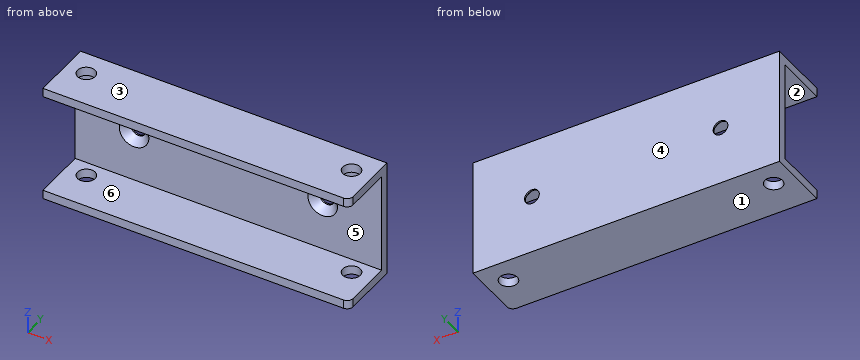
```python
from build123d import *

# Parameters (mm, degrees)
F0_W     = 104
F0_H     = 3
F1_DEPTH = 21
F0_H_2   = 34
F0_R     = 2.5
F2_DEPTH = 3
F4_D     = 6
F5_SIZE  = 2.5
F6_SIZE  = 2.5
F7_R     = 2


with BuildPart() as f1:
    # F0 (on Front) → F1 (new body)
    with BuildSketch(Plane.XZ):
        with Locations((0, 18.5)):
            Rectangle(F0_W, F0_H)
    extrude(amount=F1_DEPTH)



with BuildPart() as f1b:
    # F0 (on Front) → F1, piece 2 (new body)
    with BuildSketch(Plane.XZ):
        with Locations((0, -18.5)):
            Rectangle(F0_W, F0_H)
    extrude(amount=F1_DEPTH)


with BuildPart() as f1_1:
    add(f1.part)

    add(f1b.part)  # F2 merges F1b
    # F0 (on Front) → F2 (join)
    with BuildSketch(Plane.XZ):
        Rectangle(F0_W, F0_H_2)
        with Locations((-32, 0)):
            Circle(F0_R, mode=Mode.SUBTRACT)
        with Locations((32, 0)):
            Circle(F0_R, mode=Mode.SUBTRACT)
    extrude(amount=F2_DEPTH)

    # F4 (through all)
    with Locations(Plane(origin=(0, 0, -20), x_dir=(1, 0, 0), z_dir=(0, 0, -1))):
        with Locations((-45, 8.3), (45, 8.2999998429)):
            Hole(F4_D / 2)

    # F5
    f5_edges = [f1_1.edges().sort_by_distance(p)[0] for p in [
        (-34.5, -3, 0),
    ]]
    chamfer(f5_edges, length=F5_SIZE)

    # F6
    f6_edges = [f1_1.edges().sort_by_distance(p)[0] for p in [
        (29.5, -3, 0),
    ]]
    chamfer(f6_edges, length=F6_SIZE)

    # F7
    f7_edges = [f1_1.edges().sort_by_distance(p)[0] for p in [
        (52, -21, -18.5),
        (52, -21, 18.5),
    ]]
    fillet(f7_edges, radius=F7_R)


solid = f1_1.part
```
Read the model definition and answer for the solid it produces. Units are mm, in the model's axes. Face numbers are marked on the shaded views. A direction names the side the tool comes from. Coordinates: 2 decimals unless noted, no trailing zeros. Write each loop counter-clockwise with the first axis right and the second up, starting at its lowest first coordinate (ties: lowest second). Pieces come first, ordered by that corner, then holes. Notation, with made-up numbers: (4, -7.5) -> (8, -7.5) arc R29 ccw to (8, 12.5) -> close; hole circle Ø4 at (-35.75, -36.5). An arc over 180 degrees is marked (long way). Return JSON: item names as keys, results as strings.
1. Determine the mould class of the marked faces 3, 4, 5 and 6 for opening direction Z: pulls with the +Z half, pulls with the -Z half, needs draft (parallel to the pull), parting line crosses it, or undercut.
Found:
{"face 3": "pulls with the +Z half", "face 4": "needs draft", "face 5": "undercut", "face 6": "undercut"}
2. A tool of negligible diameter and unlimited length cuts with its end or side. For the marked faces 1 and 2, from which of +Z, -Z, +X, -X, +Y, -Y can it reach the whole face along a straight path? Write none if from no direction.
Found:
{"face 1": "-Z, +X, -X, +Y, -Y", "face 2": "+X, -X, -Y"}
3. A cutting plane is placed at D-D (y = -14). Determine the outline of the cut face in (x, z).
Found:
{"outline": "(-52, -20) -> (52, -20) -> (52, -17) -> (-52, -17) -> close; (-52, 17) -> (52, 17) -> (52, 20) -> (-52, 20) -> close"}
4. A cutting plane is placed at C-C (x = 32). Determine the outline of the cut face in (y, z), and give its area (3 significant figures).
Found:
{"outline": "(-21, -20) -> (0, -20) -> (0, -2.5) -> (-0.5, -2.5) -> (-3, -5) -> (-3, -17) -> (-21, -17) -> close; (-21, 17) -> (-3, 17) -> (-3, 5) -> (-0.5, 2.5) -> (0, 2.5) -> (0, 20) -> (-21, 20) -> close", "area": "207 mm2"}
5. A cutting plane is placed at A-A (z = 0). Determine the outline of the cut face in (x, y), and give its area (4 significant figures).
Found:
{"outline": "(-52, -3) -> (-37, -3) -> (-34.5, -0.5) -> (-34.5, 0) -> (-52, 0) -> close; (-29.5, -0.5) -> (-27, -3) -> (27, -3) -> (29.5, -0.5) -> (29.5, 0) -> (-29.5, 0) -> close; (34.5, -0.5) -> (37, -3) -> (52, -3) -> (52, 0) -> (34.5, 0) -> close", "area": "269.5 mm2"}
6. Each of these flat-tipped pins is pushed along its axis until it touches: P1, Ø3, axis at x = 22, z = 14, coming from the -Y side; P2, Ø6.5, axis at x = 32, z = 0, coming from the -Y side. Where does it stop, or does it pass through?
Found:
{"P1": "y = -3", "P2": "y = -1.25"}
7. Find the intervals of material crossed by line 1 along Z through (x, y) = (-42.5, -5); line 2 along Y through (x, z) = (-45, 18.3); line 3 along Z through (x, y) = (32, -0.05), in increasing order. Write a range as from..to.
Found:
{"line 1": "-20..-17, 17..20", "line 2": "-21..-11.3, -5.3..0", "line 3": "-20..-2.5, 2.5..20"}
8. A cutting plane is placed at B-B (y = -8.3). Determine the outline of the cut face in (x, z).
Found:
{"outline": "(-52, -20) -> (-48, -20) -> (-48, -17) -> (-52, -17) -> close; (-52, 17) -> (-48, 17) -> (-48, 20) -> (-52, 20) -> close; (-42, -20) -> (42, -20) -> (42, -17) -> (-42, -17) -> close; (-42, 17) -> (42, 17) -> (42, 20) -> (-42, 20) -> close; (48, -20) -> (52, -20) -> (52, -17) -> (48, -17) -> close; (48, 17) -> (52, 17) -> (52, 20) -> (48, 20) -> close"}
